Autodesk Inventor part; units mm, degrees
ref_plane "YZ Plane" through (0, 0, 0) normal (1, 0, 0) x (0, 1, 0)
ref_plane "XZ Plane" through (0, 0, 0) normal (0, 1, 0) x (-1, 0, 0)
ref_plane "XY Plane" through (0, 0, 0) normal (0, 0, 1) x (1, 0, 0)
sketch "Sketch1" plane through (0, 0, 0) normal (0, 0, 1) x (1, 0, 0)
  arc A0 (-1.0546, 0.6324) -> (-0.3475, 0.9253) centre (-1.0546, 1.6324) ccw
  line L0 (-1.0546, 0.6324) -> (-1.8676, 0.6324)
  arc A1 (-2.0676, 0.8324) -> (-1.8676, 0.6324) centre (-1.8676, 0.8324) ccw
  line L1 (-2.0676, 0.8324) -> (-2.0676, 2.6024)
  arc A2 (-2.0676, 2.6024) -> (-2.3176, 2.8524) centre (-2.3176, 2.6024) ccw
  line L2 (-2.3176, 2.8524) -> (-3.5676, 2.8524)
  arc A3 (-3.5676, 2.8524) -> (-4.0676, 2.3524) centre (-3.5676, 2.3524) ccw
  line L3 (-4.0676, 2.3524) -> (-4.0676, -2.5676)
  arc A4 (-4.0676, -2.5676) -> (-2.5676, -4.0676) centre (-2.5676, -2.5676) ccw
  line L4 (-2.5676, -4.0676) -> (2.3524, -4.0676)
  arc A5 (2.3524, -4.0676) -> (2.8524, -3.5676) centre (2.3524, -3.5676) ccw
  line L5 (2.8524, -3.5676) -> (2.8524, -2.3176)
  arc A6 (2.8524, -2.3176) -> (2.6024, -2.0676) centre (2.6024, -2.3176) ccw
  line L6 (2.6024, -2.0676) -> (0.8324, -2.0676)
  arc A7 (0.6324, -1.8676) -> (0.8324, -2.0676) centre (0.8324, -1.8676) ccw
  line L7 (0.6324, -1.8676) -> (0.6324, -1.0546)
  arc A8 (0.9253, -0.3475) -> (0.6324, -1.0546) centre (1.6324, -1.0546) ccw
  line L8 (0.9253, -0.3475) -> (4.0676, 2.7948)
  arc A9 (4.0676, 2.7948) -> (5.6798, 2.2912) centre (5.9324, 5.9324) ccw
  line L9 (5.6798, 2.2912) -> (5.9324, 2.491)
  line L10 (5.9324, 2.491) -> (6.1851, 2.2912)
  arc A10 (6.1851, 2.2912) -> (7.7973, 2.7948) centre (5.9324, 5.9324) ccw
  line L11 (7.7973, 2.7948) -> (10.9395, -0.3475)
  arc A11 (11.2324, -1.0546) -> (10.9395, -0.3475) centre (10.2324, -1.0546) ccw
  line L12 (11.2324, -1.0546) -> (11.2324, -1.8676)
  arc A12 (11.0324, -2.0676) -> (11.2324, -1.8676) centre (11.0324, -1.8676) ccw
  line L13 (11.0324, -2.0676) -> (9.2624, -2.0676)
  arc A13 (9.2624, -2.0676) -> (9.0124, -2.3176) centre (9.2624, -2.3176) ccw
  line L14 (9.0124, -2.3176) -> (9.0124, -3.5676)
  arc A14 (9.0124, -3.5676) -> (9.5124, -4.0676) centre (9.5124, -3.5676) ccw
  line L15 (9.5124, -4.0676) -> (14.4324, -4.0676)
  arc A15 (14.4324, -4.0676) -> (15.9324, -2.5676) centre (14.4324, -2.5676) ccw
  line L16 (15.9324, -2.5676) -> (15.9324, 2.3524)
  arc A16 (15.9324, 2.3524) -> (15.4324, 2.8524) centre (15.4324, 2.3524) ccw
  line L17 (15.4324, 2.8524) -> (14.1824, 2.8524)
  arc A17 (14.1824, 2.8524) -> (13.9324, 2.6024) centre (14.1824, 2.6024) ccw
  line L18 (13.9324, 2.6024) -> (13.9324, 0.8324)
  arc A18 (13.7324, 0.6324) -> (13.9324, 0.8324) centre (13.7324, 0.8324) ccw
  line L19 (13.7324, 0.6324) -> (12.9194, 0.6324)
  arc A19 (12.2123, 0.9253) -> (12.9194, 0.6324) centre (12.9194, 1.6324) ccw
  line L20 (12.2123, 0.9253) -> (9.0701, 4.0676)
  arc A20 (9.0701, 4.0676) -> (9.5737, 5.6798) centre (5.9324, 5.9324) ccw
  line L21 (9.5737, 5.6798) -> (9.3739, 5.9324)
  line L22 (9.3739, 5.9324) -> (9.5739, 6.1824)
  arc A21 (9.5739, 6.1824) -> (9.0701, 7.7973) centre (5.9324, 5.9324) ccw
  line L23 (9.0701, 7.7973) -> (12.2123, 10.9395)
  arc A22 (12.9194, 11.2324) -> (12.2123, 10.9395) centre (12.9194, 10.2324) ccw
  line L24 (12.9194, 11.2324) -> (13.7324, 11.2324)
  arc A23 (13.9324, 11.0324) -> (13.7324, 11.2324) centre (13.7324, 11.0324) ccw
  line L25 (13.9324, 11.0324) -> (13.9324, 9.2624)
  arc A24 (13.9324, 9.2624) -> (14.1824, 9.0124) centre (14.1824, 9.2624) ccw
  line L26 (14.1824, 9.0124) -> (15.4324, 9.0124)
  arc A25 (15.4324, 9.0124) -> (15.9324, 9.5124) centre (15.4324, 9.5124) ccw
  line L27 (15.9324, 9.5124) -> (15.9324, 14.4324)
  arc A26 (15.9324, 14.4324) -> (14.4324, 15.9324) centre (14.4324, 14.4324) ccw
  line L28 (14.4324, 15.9324) -> (9.5124, 15.9324)
  arc A27 (9.5124, 15.9324) -> (9.0124, 15.4324) centre (9.5124, 15.4324) ccw
  line L29 (9.0124, 15.4324) -> (9.0124, 14.1824)
  arc A28 (9.0124, 14.1824) -> (9.2624, 13.9324) centre (9.2624, 14.1824) ccw
  line L30 (9.2624, 13.9324) -> (11.0324, 13.9324)
  arc A29 (11.2324, 13.7324) -> (11.0324, 13.9324) centre (11.0324, 13.7324) ccw
  line L31 (11.2324, 13.7324) -> (11.2324, 12.9194)
  arc A30 (10.9395, 12.2123) -> (11.2324, 12.9194) centre (10.2324, 12.9194) ccw
  line L32 (10.9395, 12.2123) -> (7.7973, 9.0701)
  arc A31 (7.7973, 9.0701) -> (6.1824, 9.5739) centre (5.9324, 5.9324) ccw
  line L33 (6.1824, 9.5739) -> (5.9324, 9.3739)
  line L34 (5.9324, 9.3739) -> (5.6824, 9.5739)
  arc A32 (5.6824, 9.5739) -> (4.0676, 9.0701) centre (5.9324, 5.9324) ccw
  line L35 (4.0676, 9.0701) -> (0.9253, 12.2123)
  arc A33 (0.6324, 12.9194) -> (0.9253, 12.2123) centre (1.6324, 12.9194) ccw
  line L36 (0.6324, 12.9194) -> (0.6324, 13.7324)
  arc A34 (0.8324, 13.9324) -> (0.6324, 13.7324) centre (0.8324, 13.7324) ccw
  line L37 (0.8324, 13.9324) -> (2.6024, 13.9324)
  arc A35 (2.6024, 13.9324) -> (2.8524, 14.1824) centre (2.6024, 14.1824) ccw
  line L38 (2.8524, 14.1824) -> (2.8524, 15.4324)
  arc A36 (2.8524, 15.4324) -> (2.3524, 15.9324) centre (2.3524, 15.4324) ccw
  line L39 (2.3524, 15.9324) -> (-2.5676, 15.9324)
  arc A37 (-2.5676, 15.9324) -> (-4.0676, 14.4324) centre (-2.5676, 14.4324) ccw
  line L40 (-4.0676, 14.4324) -> (-4.0676, 9.5124)
  arc A38 (-4.0676, 9.5124) -> (-3.5676, 9.0124) centre (-3.5676, 9.5124) ccw
  line L41 (-3.5676, 9.0124) -> (-2.3176, 9.0124)
  arc A39 (-2.3176, 9.0124) -> (-2.0676, 9.2624) centre (-2.3176, 9.2624) ccw
  line L42 (-2.0676, 9.2624) -> (-2.0676, 11.0324)
  arc A40 (-1.8676, 11.2324) -> (-2.0676, 11.0324) centre (-1.8676, 11.0324) ccw
  line L43 (-1.8676, 11.2324) -> (-1.0546, 11.2324)
  arc A41 (-0.3475, 10.9395) -> (-1.0546, 11.2324) centre (-1.0546, 10.2324) ccw
  line L44 (-0.3475, 10.9395) -> (2.7948, 7.7973)
  arc A42 (2.7948, 7.7973) -> (2.291, 6.1824) centre (5.9324, 5.9324) ccw
  line L45 (2.291, 6.1824) -> (2.491, 5.9324)
  line L46 (2.491, 5.9324) -> (2.2912, 5.6798)
  arc A43 (2.2912, 5.6798) -> (2.7948, 4.0676) centre (5.9324, 5.9324) ccw
  line L47 (2.7948, 4.0676) -> (-0.3475, 0.9253)
  circle A44 centre (5.9324, 5.9324) radius 2.5
  line L48 (-1.0546, 11.0324) -> (-1.8676, 11.0324)
  line L49 (-1.8676, 11.0324) -> (-1.8676, 9.2624)
  arc A45 (-2.3176, 8.8124) -> (-1.8676, 9.2624) centre (-2.3176, 9.2624) ccw
  line L50 (-2.3176, 8.8124) -> (-3.5676, 8.8124)
  arc A46 (-4.2676, 9.5124) -> (-3.5676, 8.8124) centre (-3.5676, 9.5124) ccw
  line L51 (-4.2676, 9.5124) -> (-4.2676, 14.4324)
  arc A47 (-2.5676, 16.1324) -> (-4.2676, 14.4324) centre (-2.5676, 14.4324) ccw
  line L52 (-2.5676, 16.1324) -> (2.3524, 16.1324)
  arc A48 (3.0524, 15.4324) -> (2.3524, 16.1324) centre (2.3524, 15.4324) ccw
  line L53 (3.0524, 15.4324) -> (3.0524, 14.1824)
  arc A49 (2.6024, 13.7324) -> (3.0524, 14.1824) centre (2.6024, 14.1824) ccw
  line L54 (2.6024, 13.7324) -> (0.8324, 13.7324)
  line L55 (0.8324, 13.7324) -> (0.8324, 12.9194)
  arc A50 (0.8324, 12.9194) -> (1.0667, 12.3537) centre (1.6324, 12.9194) ccw
  line L56 (1.0667, 12.3537) -> (4.1014, 9.3191)
  arc A51 (5.7474, 9.778) -> (4.1014, 9.3191) centre (5.9324, 5.9324) ccw
  line L57 (5.7474, 9.778) -> (5.9324, 9.63)
  line L58 (5.9324, 9.63) -> (6.1174, 9.778)
  arc A52 (7.7635, 9.3191) -> (6.1174, 9.778) centre (5.9324, 5.9324) ccw
  line L59 (7.7635, 9.3191) -> (10.7981, 12.3537)
  arc A53 (10.7981, 12.3537) -> (11.0324, 12.9194) centre (10.2324, 12.9194) ccw
  line L60 (11.0324, 12.9194) -> (11.0324, 13.7324)
  line L61 (11.0324, 13.7324) -> (9.2624, 13.7324)
  arc A54 (8.8124, 14.1824) -> (9.2624, 13.7324) centre (9.2624, 14.1824) ccw
  line L62 (8.8124, 14.1824) -> (8.8124, 15.4324)
  arc A55 (9.5124, 16.1324) -> (8.8124, 15.4324) centre (9.5124, 15.4324) ccw
  line L63 (9.5124, 16.1324) -> (14.4324, 16.1324)
  arc A56 (16.1324, 14.4324) -> (14.4324, 16.1324) centre (14.4324, 14.4324) ccw
  line L64 (16.1324, 14.4324) -> (16.1324, 9.5124)
  arc A57 (15.4324, 8.8124) -> (16.1324, 9.5124) centre (15.4324, 9.5124) ccw
  line L65 (15.4324, 8.8124) -> (14.1824, 8.8124)
  arc A58 (13.7324, 9.2624) -> (14.1824, 8.8124) centre (14.1824, 9.2624) ccw
  line L66 (13.7324, 9.2624) -> (13.7324, 11.0324)
  line L67 (13.7324, 11.0324) -> (12.9194, 11.0324)
  arc A59 (12.9194, 11.0324) -> (12.3537, 10.7981) centre (12.9194, 10.2324) ccw
  line L68 (12.3537, 10.7981) -> (9.3191, 7.7635)
  arc A60 (9.778, 6.1174) -> (9.3191, 7.7635) centre (5.9324, 5.9324) ccw
  line L69 (9.778, 6.1174) -> (9.6294, 5.9317)
  line L70 (9.6294, 5.9317) -> (9.7778, 5.7441)
  arc A61 (9.3191, 4.1014) -> (9.7778, 5.7441) centre (5.9324, 5.9324) ccw
  line L71 (9.3191, 4.1014) -> (12.3537, 1.0667)
  arc A62 (12.3537, 1.0667) -> (12.9194, 0.8324) centre (12.9194, 1.6324) ccw
  line L72 (12.9194, 0.8324) -> (13.7324, 0.8324)
  line L73 (13.7324, 0.8324) -> (13.7324, 2.6024)
  arc A63 (14.1824, 3.0524) -> (13.7324, 2.6024) centre (14.1824, 2.6024) ccw
  line L74 (14.1824, 3.0524) -> (15.4324, 3.0524)
  arc A64 (16.1324, 2.3524) -> (15.4324, 3.0524) centre (15.4324, 2.3524) ccw
  line L75 (16.1324, 2.3524) -> (16.1324, -2.5676)
  arc A65 (14.4324, -4.2676) -> (16.1324, -2.5676) centre (14.4324, -2.5676) ccw
  line L76 (14.4324, -4.2676) -> (9.5124, -4.2676)
  arc A66 (8.8124, -3.5676) -> (9.5124, -4.2676) centre (9.5124, -3.5676) ccw
  line L77 (8.8124, -3.5676) -> (8.8124, -2.3176)
  arc A67 (9.2624, -1.8676) -> (8.8124, -2.3176) centre (9.2624, -2.3176) ccw
  line L78 (9.2624, -1.8676) -> (11.0324, -1.8676)
  line L79 (11.0324, -1.8676) -> (11.0324, -1.0546)
  arc A68 (11.0324, -1.0546) -> (10.7981, -0.4889) centre (10.2324, -1.0546) ccw
  line L80 (10.7981, -0.4889) -> (7.7635, 2.5457)
  arc A69 (6.1208, 2.087) -> (7.7635, 2.5457) centre (5.9324, 5.9324) ccw
  line L81 (6.1208, 2.087) -> (5.9324, 2.236)
  line L82 (5.9324, 2.236) -> (5.7441, 2.087)
  arc A70 (4.1014, 2.5457) -> (5.7441, 2.087) centre (5.9324, 5.9324) ccw
  line L83 (4.1014, 2.5457) -> (1.0667, -0.4889)
  arc A71 (1.0667, -0.4889) -> (0.8324, -1.0546) centre (1.6324, -1.0546) ccw
  line L84 (0.8324, -1.0546) -> (0.8324, -1.8676)
  line L85 (0.8324, -1.8676) -> (2.6024, -1.8676)
  arc A72 (3.0524, -2.3176) -> (2.6024, -1.8676) centre (2.6024, -2.3176) ccw
  line L86 (3.0524, -2.3176) -> (3.0524, -3.5676)
  arc A73 (2.3524, -4.2676) -> (3.0524, -3.5676) centre (2.3524, -3.5676) ccw
  line L87 (2.3524, -4.2676) -> (-2.5676, -4.2676)
  arc A74 (-4.2676, -2.5676) -> (-2.5676, -4.2676) centre (-2.5676, -2.5676) ccw
  line L88 (-4.2676, -2.5676) -> (-4.2676, 2.3524)
  arc A75 (-3.5676, 3.0524) -> (-4.2676, 2.3524) centre (-3.5676, 2.3524) ccw
  line L89 (-3.5676, 3.0524) -> (-2.3176, 3.0524)
  arc A76 (-1.8676, 2.6024) -> (-2.3176, 3.0524) centre (-2.3176, 2.6024) ccw
  line L90 (-1.8676, 2.6024) -> (-1.8676, 0.8324)
  line L91 (-1.8676, 0.8324) -> (-1.0546, 0.8324)
  arc A77 (-1.0546, 0.8324) -> (-0.4889, 1.0667) centre (-1.0546, 1.6324) ccw
  line L92 (-0.4889, 1.0667) -> (2.5457, 4.1014)
  arc A78 (2.087, 5.7441) -> (2.5457, 4.1014) centre (5.9324, 5.9324) ccw
  line L93 (2.087, 5.7441) -> (2.2354, 5.9317)
  line L94 (2.2354, 5.9317) -> (2.0869, 6.1174)
  arc A79 (2.5457, 7.7635) -> (2.0869, 6.1174) centre (5.9324, 5.9324) ccw
  line L95 (2.5457, 7.7635) -> (-0.4889, 10.7981)
  arc A80 (-0.4889, 10.7981) -> (-1.0546, 11.0324) centre (-1.0546, 10.2324) ccw
  line L96 (-4.2676, -4.2676) -> (-6.2676, -4.2676)
  line L97 (-6.2676, -4.2676) -> (-6.2676, 18.1324)
  line L98 (-6.2676, 18.1324) -> (18.1324, 18.1324)
  line L99 (18.1324, 18.1324) -> (18.1324, -4.2676)
  line L100 (18.1324, -4.2676) -> (14.4324, -4.2676)
  line L101 (-4.2676, -4.2676) -> (-2.5676, -4.2676)
  line L102 (5.9324, 5.9324) -> (1.9324, 5.9324) construction
  line L103 (1.9324, 8.3768) -> (1.9324, 3.4881)
  line L104 (9.9324, 8.3768) -> (9.9324, 3.4881)
  line L105 (8.3768, 9.9324) -> (3.4881, 9.9324)
  line L106 (5.9324, 5.9324) -> (5.9324, 9.9324) construction
  point P0 (0, 0)
  dimension "d0" = 0.2
  dimension "d1" = 2
  dimension "d2" = 22.4
  dimension "d3" = 24.4
  dimension "d4" = 4
  dimension "d5" = 4
extrude "Extrusion1" add sketch "Sketch1" along normal blind 20 contours A80 L95 L103 L92 A77 L91 L90 A76 L89 A75 L88 A74 L101 L96 L97 L98 L99 L100 A65 L75 A64 L74 A63 L73 L72 A62 L71 L104 L68 A59 L67 L66 A58 L65 A57 L64 A56 L63 A55 L62 A54 L61 L60 A53 L59 L105 L56 A50 L55 L54 A49 L53 A48 L52 A47 L51 A46 L50 A45 L49 L48
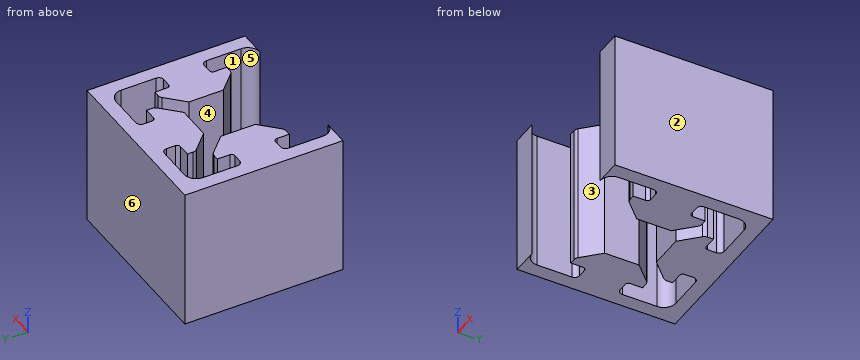
Here's how the part is built. I have some questions about the finished solid (model axes, mm). Face numbers are marked on the shaded views. A direction names the side the tool comes from. Round coordinates to 2 decimals unless told otherwise and drop trailing zeros. Order: outer loops, then holes, each group sorted by start corner. A loop starts at its lowest first (then second) coordinate and runs counter-clockwise, first axis right, second up. Notation, with made-up numbers: M -23,7 L -4,7 A30 cw -4,32 Z; hole C 73.5,67.5 d2. An arc over 180 degrees is marked long. Return JSON: item names as keys, results as strings. Group by question number.
1. If we section it at B-B on x = 15: List the corners of the cut face in (y, z) for me, then the cut area to 3 significant figures.
2. If we section it at C-C on y = 6.5: List the corners of the cut face in (x, z) for me.
3. If we section it at A-A on y = 2: List the corners of the cut face in (x, z) for me, then the cut area to 3 significant figures.
4. If we section it at D-D on y = 12: List the corners of the cut face in (x, z) for me, then the cut area to 3 significant figures.
5. I'm going to push flat-ended pins straight in: pin 1 Ø0.7 at (x, z) = (-1.5, 14) entering from -Y; pin 2 Ø2.5 at (x, z) = (11, 11) entering from -Y. Where does each tip first touch, or does it pass through?
6. Please list where these lines run through material, in increasing order: probe 1 along X at (y, z) = (4.25, 17.5); probe 2 along X at (y, z) = (9, 5.5); probe 3 along X at (y, z) = (0.25, 11.75).
7. If we mould it in two halves opening along Y, with no side actions, what happens to the marked faces 4, 5 and 6? For each: pulls with the +Y half, pulls with the -Y half, needs draft (parallel to the pull), parting line crosses it, or undercut.
8. On a 3-axis mill with a long thin cutter (end or side, diameter ignored), from which of +Z, -Z, +X, -X, +Y, -Y can I reach the whole of each face in a straight line? I mean the marked faces 1, 2 and 3. Say none if no direction works.
Reply:
{
 "1": {"outline": "M -4.27,0 L -4.17,0 L -4.17,20 L -4.27,20 Z; M 3.05,0 L 8.81,0 L 8.81,20 L 3.05,20 Z; M 16.03,0 L 18.13,0 L 18.13,20 L 16.03,20 Z", "area": "159 mm^2"},
 "2": {"outline": "M -6.27,0 L 1.93,0 L 1.93,20 L -6.27,20 Z; M 9.93,0 L 18.13,0 L 18.13,20 L 9.93,20 Z"},
 "3": {"outline": "M -6.27,0 L -4.27,0 L -4.27,20 L -6.27,20 Z; M -1.87,0 L 0.44,0 L 0.44,20 L -1.87,20 Z; M 11.42,0 L 13.73,0 L 13.73,20 L 11.42,20 Z; M 16.13,0 L 18.13,0 L 18.13,20 L 16.13,20 Z", "area": "172 mm^2"},
 "4": {"outline": "M -6.27,0 L -4.27,0 L -4.27,20 L -6.27,20 Z; M 1.42,0 L 10.44,0 L 10.44,20 L 1.42,20 Z; M 16.13,0 L 18.13,0 L 18.13,20 L 16.13,20 Z", "area": "260 mm^2"},
 "5": {"pin 1": "y = 0.83", "pin 2": "y = 1.17"},
 "6": {"probe 1": "-6.27 to 1.93, 9.93 to 18.13", "probe 2": "-6.27 to -4.04, -1.95 to 1.31, 10.56 to 13.82, 15.91 to 18.13", "probe 3": "-6.27 to -4.27, 16.13 to 18.13"},
 "7": {"face 4": "needs draft", "face 5": "undercut", "face 6": "pulls with the +Y half"},
 "8": {"face 1": "+Z, -Z", "face 2": "+Z, -Z, +X, +Y, -Y", "face 3": "+Z, -Z, -Y"}
}
